The model under review builds one solid part; all positions refer to its coordinate system, in mm. Round coordinates to 2 decimals unless told otherwise and drop trailing zeros. Write each loop counter-clockwise with the first axis right and the second up, starting at its lowest first coordinate (ties: lowest second). Pieces come first, ordered by that corner, then holes. Notation, with made-up numbers: (76, 20.25) - (118, 20.25) arc R16 cw to (118, 47.25) - close; hole circle Ø9 at (51.5, 33.5). An arc over 180 degrees is marked (long way). Return JSON: item names as keys, results as strings.
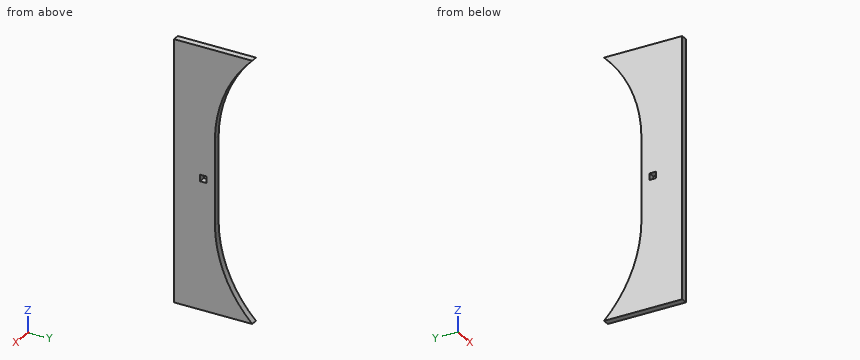
from build123d import *

# Parameters (mm, degrees)
SKETCH1_W           = 6.35
SKETCH1_H           = 6.35
BOSS_EXTRUDE1_DEPTH = 6.35


with BuildPart() as part:
    # Sketch1 → Boss-Extrude1 (new body)
    with BuildSketch(Plane(origin=(0, 0, 0), x_dir=(0, 0, -1), z_dir=(1, 0, 0))):
        with BuildLine():
            Line((-42, 1.711410462), (42, 1.711410462))
            ThreePointArc((42, 1.711410462), (88.07418015, 11.556788259), (127, 38.1))
            Line((127, 38.1), (127, -38.1))
            Line((127, -38.1), (-127, -38.1))
            Line((-127, -38.1), (-127, 38.1))
            ThreePointArc((-127, 38.1), (-88.07418015, 11.556788259), (-42, 1.711410462))
        make_face()
        with Locations((0, -9.525)):
            Rectangle(SKETCH1_W, SKETCH1_H, mode=Mode.SUBTRACT)
    extrude(amount=BOSS_EXTRUDE1_DEPTH)


solid = part.part
(1) Add section C-C (z = -13). Write out the cut boundary in (x, y), plus the area to 3 significant figures.
Filled in:
{"outline": "(0, -38.1) - (6.35, -38.1) - (6.35, 1.71) - (0, 1.71) - close", "area": "253 mm2"}
(2) Clearance check with a flat-ended pin moving along its axis: pin 1 Ø1.9 at (x, z) = (2.5, -0.5) entering from +Y. State where the tip first meets the part, or that it passes through.
Filled in:
{"pin 1": "stops at y = 1.71"}
(3) Add section B-B (y = 20). Write out the cut boundary in (x, z), plus the area to 3 significant figures.
Filled in:
{"outline": "(0, -127) - (6.35, -127) - (6.35, -104.31) - (0, -104.31) - close; (0, 104.31) - (6.35, 104.31) - (6.35, 127) - (0, 127) - close", "area": "288 mm2"}
(4) Add section A-A (x = 1.5). Write out the cut boundary in (y, z) (3 decimals), plus the area to 3 significant figures.
Filled in:
{"outline": "(-38.1, -127) - (38.1, -127) arc R122.209 cw to (1.711, -42) - (1.711, 42) arc R122.209 cw to (38.1, 127) - (-38.1, 127) - close; hole (-12.7, -3.175) - (-6.35, -3.175) - (-6.35, 3.175) - (-12.7, 3.175) - close", "area": "12,000 mm2"}
(5) Wall thickness on line 1 (Z direction, x = 4, y = 13.5); line 2 (Y direction, x = 1.75, z = 18.5); line 3 (Z direction, x = 3.25, y = 18.5): over which ranges is each line inside the solid? List them lowest first.
Filled in:
{"line 1": "z = -127 to -92.38, 92.38 to 127", "line 2": "y = -38.1 to 1.71", "line 3": "z = -127 to -101.83, 101.83 to 127"}
(6) Add section D-D (z = 55). Write out the cut boundary in (x, y).
Filled in:
{"outline": "(0, -38.1) - (6.35, -38.1) - (6.35, 2.62) - (0, 2.62) - close"}
